Source: CAD feature listing. Evaluate the final solid. Frame: model axes, mm. A direction names the side the tool comes from. Round coordinates to 2 decimals unless told otherwise and drop trailing zeros. Write each loop counter-clockwise with the first axis right and the second up, starting at its lowest first coordinate (ties: lowest second). Pieces come first, ordered by that corner, then holes. Notation, with made-up numbers: M 86,59 L 95,59 A26 cw 95,87 Z; hole C -24.5,89 d4. An arc over 180 degrees is marked long. Use a Markdown table: item, result.
```python
from build123d import *

# Parameters (mm, degrees)
SKETCH1_W                = 200
SKETCH1_H                = 150
BOSS_EXTRUDE1_DEPTH      = 15
SKETCH1_5_W              = 200
SKETCH1_5_H              = 10
REVOLVE1_ANGLE           = 90
BOSS_EXTRUDE3_REACH      = 197.256
BOSS_EXTRUDE3_END_RADIUS = 140
SKETCH1_6_W              = 10
SKETCH1_6_H              = 10
CUT_EXTRUDE2_DEPTH       = 103
CUT_EXTRUDE3_DEPTH       = 20
CUT_LOFT8_START          = -65
CUT_LOFT8_DEPTH          = 130
CUT_LOFT8_START_2        = -100
CUT_LOFT8_2_DEPTH        = 200
BOSS_EXTRUDE5_DEPTH      = 100
BOSS_EXTRUDE6_START      = -8
BOSS_EXTRUDE6_DEPTH      = 8
BOSS_EXTRUDE7_START      = -5
BOSS_EXTRUDE7_DEPTH      = 5


with BuildPart() as part:
    # Sketch1 → Boss-Extrude1 (new body)
    with BuildSketch(Plane(origin=(0, 0, 0), x_dir=(1, 0, 0), z_dir=(0, 1, 0))):
        Rectangle(SKETCH1_W, SKETCH1_H)
    extrude(amount=-BOSS_EXTRUDE1_DEPTH)

    # Sketch1<5> → Revolve1 (revolve)
    with BuildSketch(Plane(origin=(0, 0, 0), x_dir=(1, 0, 0), z_dir=(0, 1, 0))):
        with Locations((0, 70)):
            Rectangle(SKETCH1_5_W, SKETCH1_5_H)
    revolve(axis=Axis((-100, 0, 75), (1, 0, 0)), revolution_arc=REVOLVE1_ANGLE)

    # Boss-Extrude3: up to this cylinder (the profile starts inside it)
    boss_extrude3_end = Plane(origin=(0, 0, 75), z_dir=(-1, 0, 0)) * Cylinder(BOSS_EXTRUDE3_END_RADIUS, 865.512, mode=Mode.PRIVATE)
    # Sketch1<6> → Boss-Extrude3 (add, up to the surface)
    with BuildSketch(Plane(origin=(0, 0, 0), x_dir=(1, 0, 0), z_dir=(0, 1, 0)), mode=Mode.PRIVATE) as boss_extrude3_sk1:
        with Locations((-95, -70)):
            Rectangle(SKETCH1_6_W, SKETCH1_6_H)
    boss_extrude3_tool1 = extrude(boss_extrude3_sk1.sketch, amount=BOSS_EXTRUDE3_REACH, mode=Mode.PRIVATE) & boss_extrude3_end
    add(boss_extrude3_tool1.solids().sort_by_distance((-95, 0, 70))[0])
    # Sketch1<6> → Boss-Extrude3 (add, up to the surface)
    with BuildSketch(Plane(origin=(0, 0, 0), x_dir=(1, 0, 0), z_dir=(0, 1, 0)), mode=Mode.PRIVATE) as boss_extrude3_sk2:
        with Locations((95, -70)):
            Rectangle(SKETCH1_6_W, SKETCH1_6_H)
    boss_extrude3_tool2 = extrude(boss_extrude3_sk2.sketch, amount=BOSS_EXTRUDE3_REACH, mode=Mode.PRIVATE) & boss_extrude3_end
    add(boss_extrude3_tool2.solids().sort_by_distance((95, 0, 70))[0])

    # Sketch5 → Cut-Extrude2 (cut)
    with BuildSketch(Plane.ZY.offset(80)):
        Polygon((66.095917942, 143.620915339), (31.803061543, 136.620915339), (26.803061543, 161.115812766), (61.095917942, 168.115812766), align=None)
    extrude(amount=-CUT_EXTRUDE2_DEPTH, mode=Mode.SUBTRACT)

    # Sketch6 → Cut-Extrude3 (cut)
    with BuildSketch(Plane.ZY.offset(100)):
        with BuildLine():
            Line((55, 144.203533404), (65, 144.203533404))
            ThreePointArc((65, 144.203533404), (60, 157.655), (55, 144.203533404))
        make_face()
    extrude(amount=-CUT_EXTRUDE3_DEPTH, mode=Mode.SUBTRACT)

    # Cut-Loft8: read off the stored shape, not the designer's step
    # Cut-Loft8 outline → Cut-Loft8 (cut)
    with BuildSketch(Plane.XY.offset(CUT_LOFT8_START)):
        Polygon((-100, -10), (100, 0), (-100, 0), align=None)
    extrude(amount=CUT_LOFT8_DEPTH, mode=Mode.SUBTRACT)

    # Cut-Loft8 2 outline → Cut-Loft8 2 (add)
    with BuildSketch(Plane.YZ.offset(CUT_LOFT8_START_2)):
        Polygon((0, -65), (-10.4, -13), (-12, -13), (-12, -65), align=None)
    extrude(amount=CUT_LOFT8_2_DEPTH)

    # Sketch12 → Boss-Extrude5 (add)
    with BuildSketch(Plane.ZY.offset(100)):
        with BuildLine():
            Line((-65, -15), (-65, 0))
            ThreePointArc((-65, 0), (-64.208776017, 14.863266125), (-61.84404743, 29.558529783))
            Line((-61.84404743, 29.558529783), (-72.058809043, 29.558529783))
            ThreePointArc((-72.058809043, 29.558529783), (-74.262891163, 14.852249722), (-75, 0))
            Line((-75, 0), (-75, -15))
            Line((-75, -15), (-65, -15))
        make_face()
    extrude(amount=BOSS_EXTRUDE5_DEPTH)

    # Sketch12<4> → Boss-Extrude6 (add)
    with BuildSketch(Plane.ZY.offset(100).offset(BOSS_EXTRUDE6_START)):
        with BuildLine():
            Line((-65, 0), (-15, -10))
            Line((-15, -10), (-15, 29.558529783))
            Line((-15, 29.558529783), (-61.84404743, 29.558529783))
            ThreePointArc((-61.84404743, 29.558529783), (-64.208776017, 14.863266125), (-65, 0))
        make_face()
    extrude(amount=BOSS_EXTRUDE6_DEPTH)

    # Sketch21 → Boss-Extrude7 (add)
    with BuildSketch(Plane.ZY.offset(200).offset(BOSS_EXTRUDE7_START)):
        with BuildLine():
            Line((-61.84404743, 29.558529783), (72.644533384, 29.558529783))
            Line((72.644533384, 29.558529783), (72.644533384, -15))
            Line((72.644533384, -15), (-65, -15))
            Line((-65, -15), (-65, 0))
            ThreePointArc((-65, 0), (-64.208776017, 14.863266125), (-61.84404743, 29.558529783))
        make_face()
    extrude(amount=BOSS_EXTRUDE7_DEPTH)


solid = part.part
```
Q1. First-contact query: pin 1 Ø4 at (x, z) = (-95.5, -35.5) entering from +Y; pin 2 Ø14.5 at (y, z) = (141.5, 53) entering from -X; pin 3 Ø4.5 at (x, y) = (-137.5, -7) entering from +Z; pin 4 Ø1.5 at (y, z) = (30.5, -24) entering from +X. Flat tips, straight axial feed; report the tip coordinate or a pass-through.
Results are:
| item | result |
|---|---|
| pin 1 | y = 103.57 |
| pin 2 | x = -100 |
| pin 3 | z = -65 |
| pin 4 | through |
Q2. Reachability of faces 1 (the flat face through (-165, 29.559, -64)), 2 (the flat face through (-15, -2, 65)), 3 (the flat face through (-1, 0, 70)) from +Z, -Z, +X, -X, +Y, -Y: full face, straight path, thin tool, end or side. Return the list, or none.
Results are:
| item | result |
|---|---|
| face 1 | +Z, -Z, -X, +Y |
| face 2 | none |
| face 3 | +Z |
Q3. Mould query, pull axis X, two halves, no side actions, for faces 4 (the flat face through (0, -6, 75)), 5 (the flat face through (-1.4, -5.07, 13.53)). Classes: +X half, -X half, draft (parallel to the pull), parting line (faces both ways), or undercut.
Results are:
| item | result |
|---|---|
| face 4 | draft |
| face 5 | undercut |
Q4. Section B-B on y = 57. Return loops of the section in (x, z), plus the area to 3 significant figures.
Results are:
| item | result |
|---|---|
| outline | M -100,-63.75 L 100,-63.75 L 100,-52.87 L -100,-52.87 Z; M -100,65 L -90,65 L -90,75 L -100,75 Z; M 90,65 L 100,65 L 100,75 L 90,75 Z |
| area | 2,380 mm^2 |
Q5. Section C-C on x = 81. Return loops of the section in (y, z).
Results are:
| item | result |
|---|---|
| outline | M -15,-75 L 0,-75 A150 ccw 150,75 L 140,75 A140 cw 0,-65 L -0.95,-60.25 L -0.95,65 L 0,65 L 0,75 L -15,75 Z |
Q6. Section D-D on y = 3.5. Return loops of the section in (x, z).
Results are:
| item | result |
|---|---|
| outline | M -200,-74.96 L 100,-74.96 L 100,-64.96 L -92,-64.96 L -92,-15 L -100,-15 L -100,-64.96 L -195,-64.96 L -195,72.64 L -200,72.64 Z; M -100,65 L -90,65 L -90,75 L -100,75 Z; M 90,65 L 100,65 L 100,75 L 90,75 Z |
Q7. Line query: L1, parallel to Y at x = 37.5, z = 66; L2, parallel to X at y = 15, z = -29.5; L3, parallel to Y at x = -89.5, z = -20. Output: solid intervals per line, ascending.
Results are:
| item | result |
|---|---|
| L1 | -15 to 0, 139.71 to 149.73 |
| L2 | -200 to -195, -100 to -92 |
| L3 | -15 to -9, 102.83 to 116.08 |
Q8. Section A-A on z = -53.5. Return loops of the section in (x, y).
Results are:
| item | result |
|---|---|
| outline | M -200,-15 L -195,-15 L -195,29.56 L -200,29.56 Z; M -100,-15 L 100,-15 L 100,0 L 54,-2.3 L -92,-2.3 L -92,29.56 L -100,29.56 Z; M -100,55.57 L 100,55.57 L 100,77.38 L -100,77.38 Z |
